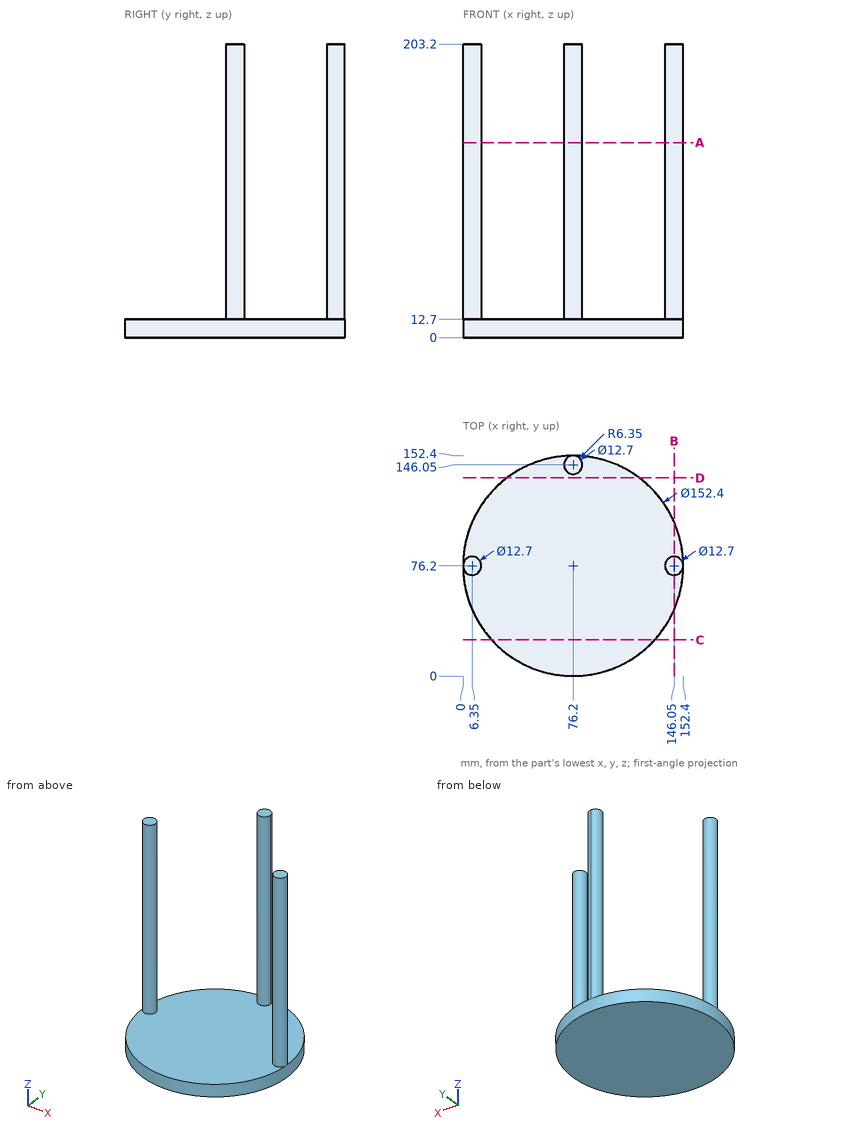
The figure shows three views and two pictorial views of one solid part (mm, origin at its lowest corner). Answer the questions. Coordinates: 2 decimals unless noted, no trailing zeros. Loops run counter-clockwise (first coordinate to the right, second up) from the corner with the lowest first, then second, coordinate; pieces in that order, holes last.
1) Find section A-A on z = 135. Write down the section's boundary in (x, y).
2) Flat-ended cylindrical pins translate along their axes: pin 1 Ø2 at (y, z) = (73, 60.5) entering from +X; pin 2 Ø5 at (x, z) = (83.5, 46) entering from +Y. Find the tip coordinate at first contact, or state that the pin passes through.
3) Find section C-C on y = 25. Write down the section's boundary in (x, z), then the cut area to 3 significant figures.
4) Find the intervals of material crossed by L1, parallel to Z at x = 40.5, y = 74; L2, parallel to Y at x = 79, z = 157; L3, parallel to Y at x = 74, z = 118.5, in increasing order.
5) Find section B-B on x = 146.05. Write down the section's boundary in (y, z), then the cut area to 3 significant figures.
6) Find section D-D on y = 137. Write down the section's boundary in (x, z), then the cut area to 3 significant figures.
Values:
1. outline: circle Ø12.7 at (6.35, 76.2); circle Ø12.7 at (76.2, 146.05); circle Ø12.7 at (146.05, 76.2)
2. pin 1: stops at x = 152.01
2. pin 2: stops at y = 150.21
3. outline: (19.76, 0) - (132.64, 0) - (132.64, 12.7) - (19.76, 12.7) - close
3. area: 1,430 mm2
4. L1: z = 0 to 12.7
4. L2: y = 140.35 to 151.75
4. L3: y = 140.09 to 152.01
5. outline: (45.75, 0) - (106.65, 0) - (106.65, 12.7) - (82.55, 12.7) - (82.55, 203.2) - (69.85, 203.2) - (69.85, 12.7) - (45.75, 12.7) - close
5. area: 3,190 mm2
6. outline: (30.27, 0) - (122.13, 0) - (122.13, 12.7) - (30.27, 12.7) - close
6. area: 1,170 mm2
